Here's the drawing with two shaded views (mm, measured from the low corner). I have some questions. Give positions to 0.01 mm unless a question says otherwise; leave off trailing zeros. Loops run counter-clockwise (first coordinate to the right, second up) from the corner with the lowest first, then second, coordinate; pieces in that order, holes last. Notation, with made-up numbers: (74.5, 1.25) - (126.5, 1.25) arc R21 cw to (126.5, 9.25) - close; hole circle Ø5 at (64, 77.25). An arc over 180 degrees is marked (long way). Answer as a JSON object with one key per item and string values. Group by question number.
Item 1: Suppose I cut it at B-B on z = 1.25. Write out the boundary of the cut face in (x, y), and give its area (3 significant figures).
Item 2: Suppose I cut it at C-C on y = 50. Write out the boundary of the cut face in (x, z), and give its area (3 significant figures).
Item 3: Please list where these lines run through material, in increasing order: L1, parallel to X at y = 10, z = 5.5; L2, parallel to Y at x = 93, z = 8.25; L3, parallel to X at y = 28, z = 7.5.
Item 4: Suppose I cut it at D-D on y = 28.5. Write out the boundary of the cut face in (x, z).
Item 5: Suppose I cut it at A-A on y = 10. Write out the boundary of the cut face in (x, z).
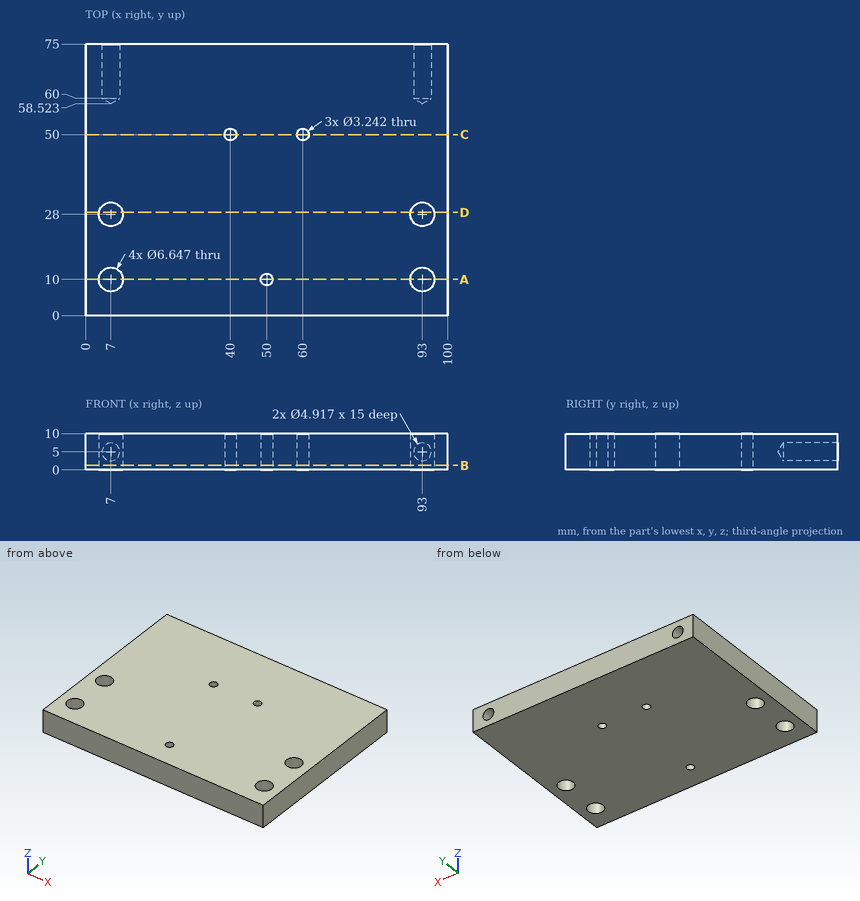
Worked out:
{
 "1": {"outline": "(0, 0) - (100, 0) - (100, 75) - (0, 75) - close; hole circle Ø6.65 at (7, 10); hole circle Ø6.65 at (7, 28); hole circle Ø3.24 at (40, 50); hole circle Ø3.24 at (50, 10); hole circle Ø3.24 at (60, 50); hole circle Ø6.65 at (93, 10); hole circle Ø6.65 at (93, 28)", "area": "7,340 mm2"},
 "2": {"outline": "(0, 0) - (38.38, 0) - (38.38, 10) - (0, 10) - close; (41.62, 0) - (58.38, 0) - (58.38, 10) - (41.62, 10) - close; (61.62, 0) - (100, 0) - (100, 10) - (61.62, 10) - close", "area": "935 mm2"},
 "3": {"L1": "x = 0 to 3.68, 10.32 to 48.38, 51.62 to 89.68, 96.32 to 100", "L2": "y = 0 to 6.68, 13.32 to 24.68, 31.32 to 75", "L3": "x = 0 to 3.68, 10.32 to 89.68, 96.32 to 100"},
 "4": {"outline": "(0, 0) - (3.71, 0) - (3.71, 10) - (0, 10) - close; (10.29, 0) - (89.71, 0) - (89.71, 10) - (10.29, 10) - close; (96.29, 0) - (100, 0) - (100, 10) - (96.29, 10) - close"},
 "5": {"outline": "(0, 0) - (3.68, 0) - (3.68, 10) - (0, 10) - close; (10.32, 0) - (48.38, 0) - (48.38, 10) - (10.32, 10) - close; (51.62, 0) - (89.68, 0) - (89.68, 10) - (51.62, 10) - close; (96.32, 0) - (100, 0) - (100, 10) - (96.32, 10) - close"}
}
